Autodesk Inventor part; units mm, degrees
ref_plane "YZ Plane" through (0, 0, 0) normal (1, 0, 0) x (0, 1, 0)
ref_plane "XZ Plane" through (0, 0, 0) normal (0, 1, 0) x (-1, 0, 0)
ref_plane "XY Plane" through (0, 0, 0) normal (0, 0, 1) x (1, 0, 0)
sketch "Esquisse1" plane through (0, 0, 0) normal (0, 0, 1) x (1, 0, 0)
  line L0 (0, 0) -> (19, 0)
  line L1 (19, 0) -> (19, 18)
  line L2 (19, 18) -> (0, 18)
  line L3 (0, 18) -> (0, 0)
  dimension "d0" = 19
  dimension "d1" = 18
extrude "Extrusion1" add sketch "Esquisse1" along normal blind 3
sketch "Esquisse2" plane through (0, 0, 3) normal (0, 0, 1) x (1, 0, 0)
  line L0 (19, 18) -> (0, 18)
  line L1 (0, 18) -> (0, 0)
  circle A0 centre (2.5, 2.5) radius 1.5
  circle A1 centre (2.5, 15.5) radius 1.5
  dimension "d4" = 13
  dimension "d5" = 2.5
  dimension "d6" = 2.5
  dimension "d7" = 2.5
  dimension "d8" = 3
  dimension "d9" = 3
extrude "Extrusion2" cut sketch "Esquisse2" against normal through all
properties part number "TOF - VL6180X Fermion SEN0427"
Geometry check sheet. Reference: the model listing, model coordinates, mm. Coordinates: 2 decimals unless noted, no trailing zeros. Order: outer loops, then holes, each group sorted by start corner. A loop starts at its lowest first (then second) coordinate and runs counter-clockwise, first axis right, second up. Notation, with made-up numbers: (42.25, 4) - (62.25, 4) arc R16 cw to (62.25, 12) - close; hole circle Ø3 at (-34, 26). An arc over 180 degrees is marked (long way). Answer in a Markdown table with one row per item. Add a question column.
1) Material ranges on line 1 along Y through (x, z) = (2.5, 2.15), recorded low to high. Write a range as [from, to].
2) Cross-section at B-B, the plane y = 1.75. Record the cut outline in (x, z), then the cut area to 3 significant figures.
3) Release check for a two-part mould opening along Y. For faces 1 (the flat face through (9, 9, 3)), 2 (the cylindrical face through (1.39, 16.51, 1.52)), 3 (the flat face through (10, 18, 1)) record: +Y half, -Y half, draft (parallel to the pull), parting line (faces both ways), or undercut.
4) Gauge pin test, flat end, axial feed: P1, Ø1.5, axis at x = 5.5, z = 2, coming from the -Y side. Record the tip position at first contact, or that the pin passes through.
5) Cross-section at A-A, the plane x = 2.5. Record the cut outline in (y, z), then the cut area to 3 significant figures.
6) Cross-section at C-C, the plane z = 0.65. Record the cut outline in (x, y).
Check result:
| question | item | result |
|---|---|---|
| 1 | line 1 | y = [0, 1], [4, 14], [17, 18] |
| 2 | outline | (0, 0) - (1.2, 0) - (1.2, 3) - (0, 3) - close; (3.8, 0) - (19, 0) - (19, 3) - (3.8, 3) - close |
| 2 | area | 49.2 mm² |
| 3 | face 1 | draft |
| 3 | face 2 | undercut |
| 3 | face 3 | +Y half |
| 4 | P1 | stops at y = 0 |
| 5 | outline | (0, 0) - (1, 0) - (1, 3) - (0, 3) - close; (4, 0) - (14, 0) - (14, 3) - (4, 3) - close; (17, 0) - (18, 0) - (18, 3) - (17, 3) - close |
| 5 | area | 36.0 mm² |
| 6 | outline | (0, 0) - (19, 0) - (19, 18) - (0, 18) - close; hole circle Ø3 at (2.5, 2.5); hole circle Ø3 at (2.5, 15.5) |
